Source: CAD feature listing. Evaluate the final solid. Frame: model axes, mm. Face numbers are marked on the shaded views. A direction names the side the tool comes from. Round coordinates to 2 decimals unless told otherwise and drop trailing zeros. Write each loop counter-clockwise with the first axis right and the second up, starting at its lowest first coordinate (ties: lowest second). Pieces come first, ordered by that corner, then holes. Notation, with made-up numbers: M 52.5,25.5 L 84.5,25.5 A14 ccw 84.5,52.5 Z; hole C 14,12 d8. An arc over 180 degrees is marked long. Use a Markdown table: item, result.
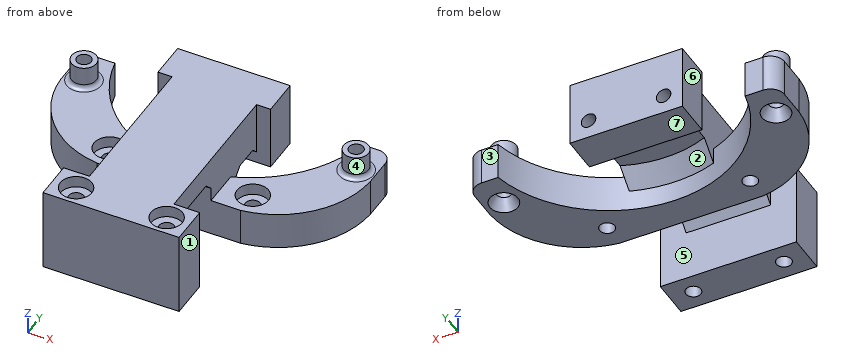
```python
from build123d import *

# Parameters (mm, degrees)
SKETCH_1_R          = 1.6
SKETCH_1_R_2        = 1.55
EXTRUDE_1_DEPTH     = 8
SKETCH_2_R          = 1.6
EXTRUDE_2_DEPTH     = 10
SKETCH_5_R          = 2.65
SKETCH_5_R_2        = 1.55
EXTRUDE_3_DEPTH     = 5
SKETCH_6_R          = 3.35
CUT_EXTRUDE_1_DEPTH = 2.5
SKETCH_13_W         = 29
SKETCH_13_H         = 8
EXTRUDE_6_DEPTH     = 8.4
SKETCH_14_R         = 1.6
CUT_EXTRUDE_4_DEPTH = 19
SKETCH_15_R         = 3.35
CUT_EXTRUDE_5_DEPTH = 2.5
EXTRUDE_7_DEPTH     = 8
SKETCH_20_R         = 1.55
CUT_EXTRUDE_7_DEPTH = 5
CHAMFER_2_SIZE      = 3.5
CHAMFER_3_SIZE      = 1.5
SKETCH_21_W         = 4.98994274
SKETCH_21_H         = 15.1
CUT_EXTRUDE_8_DEPTH = 26
CHAMFER_5_SIZE      = 2
FILLET_1_R          = 1


with BuildPart() as part:
    # 草图1 → 凸台-拉伸1 (new body)
    with BuildSketch(Plane.XY):
        with BuildLine():
            Line((-31.726131322, 22.677257125), (-31.726131322, 16.677257125))
            ThreePointArc((-31.726131322, 16.677257125), (-26.352930604, 3.872967216), (-13.976131322, -2.422742875))
            Line((-13.976131322, -2.422742875), (16.523868678, -2.422742875))
            ThreePointArc((16.523868678, -2.422742875), (28.90066796, 3.872967216), (34.273868678, 16.677257125))
            Line((34.273868678, 16.677257125), (34.273868678, 22.677257125))
            ThreePointArc((34.273868678, 22.677257125), (33.395189022, 24.798577469), (31.273868678, 25.677257125))
            Line((31.273868678, 25.677257125), (27.717127655, 25.677257125))
            ThreePointArc((27.717127655, 25.677257125), (1.404173951, 4.105735727), (-24.908779753, 25.677257125))
            Line((-24.908779753, 25.677257125), (-28.726131322, 25.677257125))
            ThreePointArc((-28.726131322, 25.677257125), (-30.847451665, 24.798577469), (-31.726131322, 22.677257125))
        make_face()
        with Locations((-13.976131322, 2.677257125)):
            Circle(SKETCH_1_R, mode=Mode.SUBTRACT)
        with Locations((16.523868678, 2.677257125)):
            Circle(SKETCH_1_R, mode=Mode.SUBTRACT)
        with Locations((30.273868678, 18.477257125)):
            Circle(SKETCH_1_R_2, mode=Mode.SUBTRACT)
        with Locations((-27.726131322, 18.477257125)):
            Circle(SKETCH_1_R_2, mode=Mode.SUBTRACT)
    extrude(amount=EXTRUDE_1_DEPTH)

    # 草图2 → 凸台-拉伸2 (add)
    with BuildSketch(Plane.XY.offset(8)):
        Polygon((-7.726131322, -17.522742875), (-11.226131322, -17.522742875), (-13.226131322, -17.522742875), (-13.226131322, -25.922742875), (-11.226131322, -25.922742875), (13.773868678, -25.922742875), (15.773868678, -25.922742875), (15.773868678, -17.522742875), (13.773868678, -17.522742875), (10.273868678, -17.522742875), (10.273868678, -2.422742875), (10.273868678, 20.927257125), (10.273868678, 24.127257125), (-7.726131322, 24.127257125), (-7.726131322, 20.927257125), (-7.726131322, -2.422742875), align=None)
        with Locations((10.923868678, -21.722742875)):
            Circle(SKETCH_2_R, mode=Mode.SUBTRACT)
        with Locations((-8.376131322, -21.722742875)):
            Circle(SKETCH_2_R, mode=Mode.SUBTRACT)
    extrude(amount=EXTRUDE_2_DEPTH)

    # 草图4 → 切除-旋转4 (revolve, cut)
    with BuildSketch(Plane(origin=(0, 18.477257125, 0), x_dir=(-1, 0, 0), z_dir=(0, -1, 0))):
        Polygon((-30.273868678, 0), (-33.273868678, 0), (-31.823868678, -2.5), (-30.273868678, -2.5), align=None)
    cut_revolve_4 = revolve(axis=Axis((30.273868678, 18.477257125, 2.5), (0, 0, 1)), mode=Mode.SUBTRACT)

    # 镜向1: 切除-旋转4 across plane
    add(cut_revolve_4.mirror(Plane(origin=(1.273868678, 0, 0), x_dir=(0, 0, 1), z_dir=(1, 0, 0))), mode=Mode.SUBTRACT)

    # 草图5 → 凸台-拉伸3 (add)
    with BuildSketch(Plane.XY.offset(8)):
        with Locations((-27.726131322, 18.477257125)):
            Circle(SKETCH_5_R)
        with Locations((-27.726131322, 18.477257125)):
            Circle(SKETCH_5_R_2, mode=Mode.SUBTRACT)
        with Locations((30.273868678, 18.477257125)):
            Circle(SKETCH_5_R)
        with Locations((30.273868678, 18.477257125)):
            Circle(SKETCH_5_R_2, mode=Mode.SUBTRACT)
    extrude(amount=EXTRUDE_3_DEPTH)

    # 草图6 → 切除-拉伸1 (cut)
    with BuildSketch(Plane.XY.offset(8)):
        with Locations((-13.976131322, 2.677257125)):
            Circle(SKETCH_6_R)
        with Locations((16.523868678, 2.677257125)):
            Circle(SKETCH_6_R)
    extrude(amount=-CUT_EXTRUDE_1_DEPTH, mode=Mode.SUBTRACT)

    # 草图13 → 凸台-拉伸6 (add)
    with BuildSketch(Plane.XZ.offset(25.922742875)):
        with Locations((1.273868678, 4)):
            Rectangle(SKETCH_13_W, SKETCH_13_H)
    extrude(amount=-EXTRUDE_6_DEPTH)

    # 草图14 → 切除-拉伸4 (cut, through all)
    with BuildSketch(Plane(origin=(0, 0, 0), x_dir=(-1, 0, 0), z_dir=(0, 0, -1))):
        with Locations((-10.923868678, -21.722742875)):
            Circle(SKETCH_14_R)
        with Locations((8.376131322, -21.722742875)):
            Circle(SKETCH_14_R)
    extrude(amount=-CUT_EXTRUDE_4_DEPTH, mode=Mode.SUBTRACT)

    # 草图15 → 切除-拉伸5 (cut)
    with BuildSketch(Plane.XY.offset(18)):
        with Locations((-8.376131322, -21.722742875)):
            Circle(SKETCH_15_R)
        with Locations((10.923868678, -21.722742875)):
            Circle(SKETCH_15_R)
    extrude(amount=-CUT_EXTRUDE_5_DEPTH, mode=Mode.SUBTRACT)

    # 草图16 → 凸台-拉伸7 (add)
    with BuildSketch(Plane(origin=(0, 24.127257125, 0), x_dir=(1, 0, 0), z_dir=(0, 1, 0))):
        Polygon((-7.726131322, -18), (-10.726131322, -18), (-10.726131322, -8), (-10.726131322, -3.990704144), (13.273868678, -3.990704144), (13.273868678, -8), (13.273868678, -18), align=None)
    extrude(amount=-EXTRUDE_7_DEPTH)

    # 草图20 → 切除-拉伸7 (cut)
    with BuildSketch(Plane(origin=(0, 24.127257125, 0), x_dir=(1, 0, 0), z_dir=(0, 1, 0))):
        with Locations((-6.726131322, -8)):
            Circle(SKETCH_20_R)
        with Locations((9.273868678, -8)):
            Circle(SKETCH_20_R)
    extrude(amount=-CUT_EXTRUDE_7_DEPTH, mode=Mode.SUBTRACT)

    # 倒角2
    chamfer_2_edges = [part.edges().sort_by_distance(p)[0] for p in [
        (1.265856801, 4.10609221, 8),
    ]]
    chamfer(chamfer_2_edges, length=CHAMFER_2_SIZE)

    # 倒角3
    chamfer_3_edges = [part.edges().sort_by_distance(p)[0] for p in [
        (1.273868678, 16.127257125, 8),
    ]]
    chamfer(chamfer_3_edges, length=CHAMFER_3_SIZE)

    # 草图21 → 切除-拉伸8 (cut)
    with BuildSketch(Plane(origin=(10.273868678, 0, 0), x_dir=(0, 0, -1), z_dir=(1, 0, 0))):
        with Locations((-10.49497137, -9.972742875)):
            Rectangle(SKETCH_21_W, SKETCH_21_H)
    extrude(amount=-CUT_EXTRUDE_8_DEPTH, mode=Mode.SUBTRACT)

    # 倒角5
    chamfer_5_edges = [part.edges().sort_by_distance(p)[0] for p in [
        (1.273868678, -17.522742875, 12.98994274),
        (1.273868678, -2.422742875, 12.98994274),
    ]]
    chamfer(chamfer_5_edges, length=CHAMFER_5_SIZE)

    # 圆角1
    fillet_1_edges = [part.edges().sort_by_distance(p)[0] for p in [
        (-30.376131322, 18.477257125, 8),
        (27.623868678, 18.477257125, 8),
    ]]
    fillet(fillet_1_edges, radius=FILLET_1_R)


solid = part.part
```
Q1. Reachability of the marked faces 4, 5, 6 and 7 from +Z, -Z, +X, -X, +Y, -Y: full face, straight path, thin tool, end or side. Return the list, or none.
Results are:
| item | result |
|---|---|
| face 4 | +Z |
| face 5 | -Z |
| face 6 | +Z, -Z, +Y |
| face 7 | -Z, +Y |
Q2. Section A-A on z = 12.25. Return loops of the section in (x, y), plus the area to 3 significant figures.
Results are:
| item | result |
|---|---|
| outline | C -27.73,18.48 d5.3; M -13.23,-25.92 L 15.77,-25.92 L 15.77,-17.52 L 10.27,-17.52 L 10.27,-16.26 L -7.73,-16.26 L -7.73,-17.52 L -13.23,-17.52 Z; M -10.73,16.13 L -7.73,16.13 L -7.73,-3.68 L 10.27,-3.68 L 10.27,16.13 L 13.27,16.13 L 13.27,24.13 L -10.73,24.13 Z; C 30.27,18.48 d5.3; hole C -27.73,18.48 d3.1; hole C -8.38,-21.72 d3.2; hole C 10.92,-21.72 d3.2; hole C 30.27,18.48 d3.1 |
| area | 828 mm^2 |
Q3. Section B-B on y = -21. Return loops of the section in (x, z), plus the area to 3 significant figures.
Results are:
| item | result |
|---|---|
| outline | M -13.23,0 L -9.8,0 L -9.8,15.5 L -11.65,15.5 L -11.65,18 L -13.23,18 Z; M -6.95,0 L 9.5,0 L 9.5,15.5 L 7.65,15.5 L 7.65,18 L -5.11,18 L -5.11,15.5 L -6.95,15.5 Z; M 12.35,0 L 15.77,0 L 15.77,18 L 14.19,18 L 14.19,15.5 L 12.35,15.5 Z |
| area | 401 mm^2 |
Q4. Mould query, pull axis Y, two halves, no side actions, for the marked faces 1, 2 and 3. Classes: +Y half, -Y half, draft (parallel to the pull), parting line (faces both ways), or undercut.
Results are:
| item | result |
|---|---|
| face 1 | draft |
| face 2 | undercut |
| face 3 | +Y half |
Q5. Section C-C on x = -21. Return loops of the section in (y, z), plus the area to 3 significant figures.
Results are:
| item | result |
|---|---|
| outline | M -0.23,0 L 16.17,0 L 16.17,8 L -0.23,8 Z |
| area | 131 mm^2 |
Q6. First-contact query: pin 1 Ø12 at (x, y) = (-15, 9) entering from +Z; pin 2 Ø2 at (x, y) = (12.5, -20.5) entering from +Z; pin 3 Ø2.5 at (x, z) = (8.5, 7.5) entering from +Y; pin 4 Ø3 at (x, y) = (16.52, 2.68) entering from +Z. Flat tips, straight axial feed; report the tip coordinate or a pass-through.
Results are:
| item | result |
|---|---|
| pin 1 | z = 8 |
| pin 2 | z = 15.5 |
| pin 3 | y = 24.13 |
| pin 4 | through |
Q7. Line query: L1, parallel to Y at x = 8.5, z = 7.25; L2, parallel to X at y = 3, z = 2.25; L3, parallel to Y at x = 10, z = 10.5. Output: solid intervals per line, ascending.
Results are:
| item | result |
|---|---|
| L1 | -25.92 to -17.52, -2.42 to 7.92, 15.38 to 19.13 |
| L2 | -25.49 to -15.54, -12.41 to 14.96, 18.09 to 28.04 |
| L3 | -25.92 to -23.03, -20.42 to -17.52, -2.42 to 24.13 |
